Autodesk Inventor part; units mm, degrees
ref_plane "YZ Plane" through (0, 0, 0) normal (1, 0, 0) x (0, 1, 0)
ref_plane "XZ Plane" through (0, 0, 0) normal (0, 1, 0) x (-1, 0, 0)
ref_plane "XY Plane" through (0, 0, 0) normal (0, 0, 1) x (1, 0, 0)
sketch "草圖1" plane through (0, 0, 0) normal (0, 1, 0) x (-1, 0, 0)
  line L0 (0, 0) -> (0, -140)
  line L1 (15, -140) -> (15, 0)
  line L2 (6, 0) -> (6, 3)
  line L3 (6, 3) -> (14.1, 3)
  line L4 (14.1, 3) -> (14.1, 0)
  line L5 (15, 0) -> (14.1, 0)
  line L6 (6, 0) -> (0, 0)
  line L7 (6, -140) -> (6, -143)
  line L8 (6, -143) -> (14.1, -143)
  line L9 (14.1, -143) -> (14.1, -140)
  line L10 (0, -140) -> (6, -140)
  line L11 (14.1, -140) -> (15, -140)
  dimension "d1" = 15
  dimension "d2" = 3
  dimension "d3" = 8.1
  dimension "d4" = 6
  dimension "d5" = 3
  dimension "d6" = 140
  dimension "d7" = 6
  dimension "d8" = 8.1
  dimension "d9" = 15
  dimension "d10" = 140
extrude "擠出1" add sketch "草圖1" along normal blind 3
sketch "草圖2" plane through (0, 3, 0) normal (0, 1, 0) x (1, 0, 0)
  line L0 (-11, 1) -> (-8, 1)
  line L1 (-8, 1) -> (-8, 7)
  line L2 (-8, 7) -> (-11, 7)
  line L3 (-11, 7) -> (-11, 1)
  line L4 (0, 0) -> (0, 140)
  line L5 (-6, 0) -> (0, 0)
  line L6 (-11, 133) -> (-8, 133)
  line L7 (-8, 133) -> (-8, 139)
  line L8 (-8, 139) -> (-11, 139)
  line L9 (-11, 139) -> (-11, 133)
  line L10 (0, 140) -> (-6, 140)
  line L11 (-15, 140) -> (-15, 0)
  dimension "d13" = 6
  dimension "d14" = 3
  dimension "d16" = 1
  dimension "d17" = 6
  dimension "d18" = 3
  dimension "d20" = 1
  dimension "d33" = 4
  dimension "d34" = 4
extrude "擠出2" cut sketch "草圖2" against normal up to surface (3 mm away)
sketch "草圖4" plane through (0, 3, 0) normal (0, 1, 0) x (1, 0, 0)
  line L0 (-44, 0) -> (-15, 0)
  line L1 (-15, 0) -> (-15, 140)
  line L2 (-15, 140) -> (-44, 140)
  line L3 (-46, 138) -> (-46, 2)
  line L4 (-15, 140) -> (-15, 0)
  line L5 (0, 140) -> (-6, 140)
  line L6 (-6, 0) -> (0, 0)
  line L7 (-39, 10) -> (-39, 63) construction
  line L8 (-37, 10) -> (-37, 63)
  line L9 (-41, 63) -> (-41, 10)
  arc A0 (-41, 10) -> (-37, 10) centre (-39, 10) ccw
  arc A1 (-37, 63) -> (-41, 63) centre (-39, 63) ccw
  circle A2 centre (-39, 130) radius 2
  arc A3 (-46, 2) -> (-44, 0) centre (-44, 2) ccw
  arc A4 (-44, 140) -> (-46, 138) centre (-44, 138) ccw
  point P0 (-39, 36.5)
  dimension "d23" = 31
  dimension "d24" = 4
  dimension "d25" = 53
  dimension "d26" = 5
  dimension "d27" = 10
  dimension "d29" = 2
  dimension "d32" = 10
extrude "擠出3" add sketch "草圖4" against normal up to surface (3 mm away)
sketch "草圖6" plane through (0, 3, 0) normal (0, 1, 0) x (1, 0, 0)
  circle A0 centre (-39, 130) radius 2
  arc A1 (-41, 10) -> (-37, 10) centre (-39, 10) ccw
  line L0 (-41, 10) -> (-41, 63)
  arc A2 (-37, 63) -> (-41, 63) centre (-39, 63) ccw
  line L1 (-37, 63) -> (-37, 10)
  line L2 (-8, 7) -> (-8, 1)
  line L3 (-8, 1) -> (-11, 1)
  line L4 (-11, 1) -> (-11, 7)
  line L5 (-11, 7) -> (-8, 7)
  line L6 (-8, 133) -> (-11, 133)
  line L7 (-11, 133) -> (-11, 139)
  line L8 (-11, 139) -> (-8, 139)
  line L9 (-8, 139) -> (-8, 133)
  line L10 (0, 0) -> (0, 140)
  line L11 (0, 140) -> (-6, 140)
  line L12 (-6, 140) -> (-6, 143)
  line L13 (-6, 143) -> (-14.1, 143)
  line L14 (-14.1, 143) -> (-14.1, 140)
  line L15 (-14.1, 140) -> (-44, 140)
  arc A3 (-44, 140) -> (-46, 138) centre (-44, 138) ccw
  line L16 (-46, 138) -> (-46, 2)
  arc A4 (-46, 2) -> (-44, 0) centre (-44, 2) ccw
  line L17 (-44, 0) -> (-14.1, 0)
  line L18 (-14.1, 0) -> (-14.1, -3)
  line L19 (-14.1, -3) -> (-6, -3)
  line L20 (-6, -3) -> (-6, 0)
  line L21 (-6, 0) -> (0, 0)
  line L22 (-6, 140) -> (-6, 143)
  line L23 (-6, 0) -> (-6, 140)
extrude "擠出4" cut sketch "草圖6" against normal blind 3 contours L21 L23 L11 L10
ref_plane "工作平面1" through (-39, 3, -10) normal (1, 0, 0) x (0, 0, -1)
sketch "草圖8" plane through (0, 3, 0) normal (0, 1, 0) x (1, 0, 0)
  line L0 (-6, -3) -> (-6, 143)
  line L1 (-6, -3) -> (-20.1, -3)
  line L2 (-20.1, -3) -> (-20.1, -5)
  line L3 (-20.1, -5) -> (-6, -5)
  line L4 (-6, -5) -> (-6, -3)
  line L5 (-44, 0) -> (-14.1, 0)
  line L6 (-20.1, -5) -> (-24.1, -5)
  line L7 (-24.1, -5) -> (-24.1, 0)
  line L8 (-24.1, 0) -> (-20.1, 0)
  line L9 (-20.1, 0) -> (-20.1, -5)
  line L10 (-14.1, 0) -> (-14.1, -3)
  line L11 (-6, 143) -> (-20.1, 143)
  line L12 (-20.1, 143) -> (-20.1, 145)
  line L13 (-20.1, 145) -> (-6, 145)
  line L14 (-6, 145) -> (-6, 143)
  line L15 (-14.1, 140) -> (-44, 140)
  line L16 (-20.1, 145) -> (-24.1, 145)
  line L17 (-24.1, 145) -> (-24.1, 140)
  line L18 (-24.1, 140) -> (-20.1, 140)
  line L19 (-20.1, 140) -> (-20.1, 145)
  line L20 (-14.1, 143) -> (-14.1, 140)
  point P0 (0, 0)
  dimension "d40" = 6
  dimension "d41" = 2
  dimension "d42" = 4
  dimension "d45" = 6
  dimension "d46" = 2
  dimension "d47" = 4
extrude "擠出5" add sketch "草圖8" against normal up to surface (3 mm away) contours L11 L12 L13 L14 | L4 L3 L2 L1 | L2 L6 L7 L5 L9 | L19 L15 L17 L16 L12
sketch "草圖9" plane through (0, 3, 0) normal (0, 1, 0) x (1, 0, 0)
  line L0 (-6, -5) -> (-6, 145)
  line L1 (-6, 145) -> (-24.1, 145)
  line L2 (-24.1, 145) -> (-24.1, 140)
  line L3 (-24.1, 140) -> (-44, 140)
  arc A0 (-44, 140) -> (-46, 138) centre (-44, 138) ccw
  line L4 (-46, 138) -> (-46, 2)
  arc A1 (-46, 2) -> (-44, 0) centre (-44, 2) ccw
  line L5 (-44, 0) -> (-24.1, 0)
  line L6 (-24.1, 0) -> (-24.1, -5)
  line L7 (-24.1, -5) -> (-6, -5)
  line L8 (-14.1, -3) -> (-20.1, -3)
  line L9 (-20.1, -3) -> (-20.1, 0)
  line L10 (-20.1, 0) -> (-14.1, 0)
  line L11 (-14.1, 0) -> (-14.1, -3)
  line L12 (-20.1, 140) -> (-20.1, 143)
  line L13 (-20.1, 143) -> (-14.1, 143)
  line L14 (-14.1, 143) -> (-14.1, 140)
  line L15 (-14.1, 140) -> (-20.1, 140)
  circle A2 centre (-39, 130) radius 2
  arc A3 (-41, 10) -> (-37, 10) centre (-39, 10) ccw
  line L16 (-41, 10) -> (-41, 63)
  arc A4 (-37, 63) -> (-41, 63) centre (-39, 63) ccw
  line L17 (-37, 63) -> (-37, 10)
  line L18 (-8, 7) -> (-8, 1)
  line L19 (-8, 1) -> (-11, 1)
  line L20 (-11, 1) -> (-11, 7)
  line L21 (-11, 7) -> (-8, 7)
  line L22 (-8, 133) -> (-11, 133)
  line L23 (-11, 133) -> (-11, 139)
  line L24 (-11, 139) -> (-8, 139)
  line L25 (-8, 139) -> (-8, 133)
  point P0 (0, 0)
equation "\"d10\" = d6"
equation "\"d20\" = d16"
properties part number "chassis_1_2"
For this review, take the finished solid that the model builds, in its own axes (mm). A direction names the side the tool comes from. Coordinates: 2 decimals unless noted, no trailing zeros. Loops run counter-clockwise (first coordinate to the right, second up) from the corner with the lowest first, then second, coordinate; pieces in that order, holes last. Notation, with made-up numbers: (-9.5, 63) - (5.5, 63) arc R8 ccw to (5.5, 75) - close; hole circle Ø11 at (47, 54). An arc over 180 degrees is marked (long way). Return JSON: item names as keys, results as strings.
Item 1: For faces 4 (the flat face through (-46, 2, -71)), 5 (the flat face through (-24.1, 2, -143)), 6 (the flat face through (-34, 2, 0)), 7 (the flat face through (-8, 2, -4)), list the 3-axis set-ups (+Z, -Z, +X, -X, +Y, -Y) from which the entire face can be reached by the end or side of a thin tool; tool diameter is ignored.
Determined:
{"face 4": "+Z, -Z, -X, +Y, -Y", "face 5": "-Z, -X, +Y, -Y", "face 6": "+Z, -X, +Y, -Y", "face 7": "+Y, -Y"}
Item 2: Take a section at C-C (z = -130). Give the boundary of the cut face in (x, y).
Determined:
{"outline": "(-46, 0) - (-41, 0) - (-41, 3) - (-46, 3) - close; (-37, 0) - (-6, 0) - (-6, 3) - (-37, 3) - close"}
Item 3: Mouldability with a two-part tool opening along Z and no side actions: class faces 1 (the flat face through (-34, 2, -140)), 2 (the flat face through (-14.1, 1, 2)), 3 (the flat face through (-26, 0, -71)) as pulls with the +Z half, pulls with the -Z half, needs draft (parallel to the pull), parting line crosses it, or undercut.
Determined:
{"face 1": "pulls with the -Z half", "face 2": "undercut", "face 3": "needs draft"}
Item 4: Take a section at D-D (x = -9.5). Give the boundary of the cut face in (y, z), then the cut area to 3 significant figures.
Determined:
{"outline": "(0, -145) - (3, -145) - (3, -139) - (0, -139) - close; (0, -133) - (3, -133) - (3, -7) - (0, -7) - close; (0, -1) - (3, -1) - (3, 5) - (0, 5) - close", "area": "414 mm2"}
Item 5: Insertion check: pin 1 (0.9 mm diameter, centred on x = -33.5, y = 1.5, fed in from +Z); pin 2 (1.5 mm diameter, centred on x = -30, y = 2, fed in from -Z); pin 3 (3 mm diameter, centred on x = -39, z = -130, fed in from +Y). Each pin has a flat end and moves straight along its axis. Give the tip position at first contact, or say it passes through.
Determined:
{"pin 1": "stops at z = 0", "pin 2": "stops at z = -140", "pin 3": "passes through"}
Item 6: For line 1 (Z direction, x = -20, y = 0.8); line 2 (Z direction, x = -39, y = 2.1); line 3 (X direction, y = 2.35, z = -35), list the stretches that pass through material, from the lowest coordinate up.
Determined:
{"line 1": "z = -145 to -143, -140 to 0, 3 to 5", "line 2": "z = -140 to -132, -128 to -65, -8 to 0", "line 3": "x = -46 to -41, -37 to -6"}
Item 7: Take a section at B-B (x = -39). Give the boundary of the cut face in (y, z).
Determined:
{"outline": "(0, -140) - (3, -140) - (3, -132) - (0, -132) - close; (0, -128) - (3, -128) - (3, -65) - (0, -65) - close; (0, -8) - (3, -8) - (3, 0) - (0, 0) - close"}
Item 8: Take a section at A-A (y = 1.5). State how many separate pieces and enclosed holes the cut face has, then the cut area to 3 significant figures.
Determined:
{"separate pieces": "1", "enclosed holes": "6", "area": "5,470 mm2"}
